Read the model definition and answer for the solid it produces. Units are mm, in the model's axes. Give positions to 0.01 mm unless a question says otherwise; leave off trailing zeros. Loops run counter-clockwise (first coordinate to the right, second up) from the corner with the lowest first, then second, coordinate; pieces in that order, holes last. Notation, with made-up numbers: (55, 19.5) -> (73, 19.5) arc R24 cw to (73, 56.5) -> close; hole circle Ø9 at (3.25, 77). An arc over 180 degrees is marked (long way). Write each question's results on one line, items separated by ' | '. Start each with the question number.
Item 1: Find the intervals of material crossed by line 1 (Z direction, x = 0.1, y = -13); line 2 (Y direction, x = 0.3, z = -5.5); line 3 (Z direction, x = -0.05, y = -28), in increasing order.
Item 2: Section B-B on y = 14 is taken. Write down the section's boundary in (x, z), and give its area (3 significant figures).
Item 3: Section A-A on x = 0 is taken. Write down the section's boundary in (y, z), and give its area (3 significant figures).
Item 4: Section C-C on z = 0.25 is taken. Write down the section's boundary in (x, y).
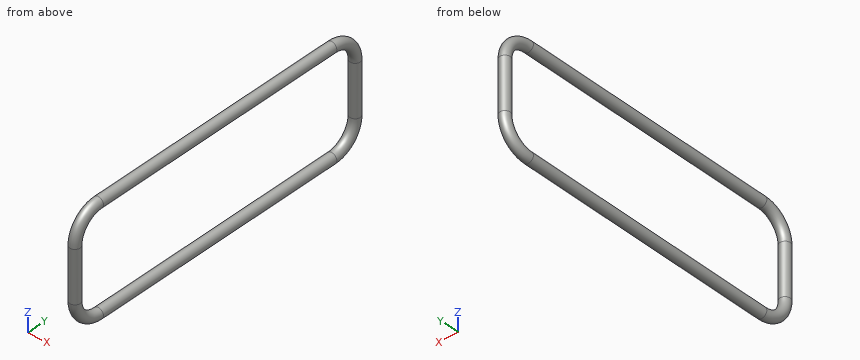
Autodesk Inventor part; units mm, degrees
ref_plane "YZ Plane" through (0, 0, 0) normal (1, 0, 0) x (0, 1, 0)
ref_plane "XZ Plane" through (0, 0, 0) normal (0, 1, 0) x (-1, 0, 0)
ref_plane "XY Plane" through (0, 0, 0) normal (0, 0, 1) x (1, 0, 0)
sketch "Sketch1" plane through (0, 0, 0) normal (1, 0, 0) x (0, 1, 0)
  line L0 (25, 10) -> (-25, 10)
  line L1 (-30, 5) -> (-30, -5)
  line L2 (-25, -10) -> (25, -10)
  line L3 (30, -5) -> (30, 5)
  line L4 (30, 10) -> (-30, -10) construction
  line L5 (-30, 10) -> (30, -10) construction
  arc A0 (30, 5) -> (25, 10) centre (25, 5) ccw
  arc A1 (25, -10) -> (30, -5) centre (25, -5) ccw
  arc A2 (-30, -5) -> (-25, -10) centre (-25, -5) ccw
  arc A3 (-25, 10) -> (-30, 5) centre (-25, 5) ccw
  point P0 (0, 0)
  dimension "d0" = 60
  dimension "d1" = 20
  dimension "d2" = 5
sketch "Sketch3" plane through (0, 0, 0) normal (0, 0, 1) x (1, 0, 0)
  circle A0 centre (0, 30) radius 1
  point P0 (0, 0)
  dimension "d4" = 2
sweep "Sweep1" add profiles "Sketch3" path "Sketch1"
properties part number "Mock String"
Findings:
1) line 1: -10.99 to -9.01, 9.01 to 10.99 | line 2: -30.93 to -29.02, 29.02 to 30.93 | line 3: -10.19 to -7.65, 7.65 to 10.19
2) outline: circle Ø2 at (0, -10); circle Ø2 at (0, 10) | area: 6.28 mm2
3) outline: (-31, -5) arc R6 ccw to (-25, -11) -> (25, -11) arc R6 ccw to (31, -5) -> (31, 5) arc R6 ccw to (25, 11) -> (-25, 11) arc R6 ccw to (-31, 5) -> close; hole (-29, -5) arc R4 ccw to (-25, -9) -> (25, -9) arc R4 ccw to (29, -5) -> (29, 5) arc R4 ccw to (25, 9) -> (-25, 9) arc R4 ccw to (-29, 5) -> close | area: 303 mm2
4) outline: circle Ø2 at (0, -30); circle Ø2 at (0, 30)
